```python
from build123d import *

# Parameters (mm, degrees)
F0_R     = 21
F0_R_2   = 0.8
F1_DEPTH = 5
F2_R     = 21
F3_DEPTH = 14
F4_R     = 21
F4_R_2   = 19
F5_DEPTH = 2.5
F6_SIZE  = 1


with BuildPart() as f1:
    # F0 (on Top) → F1 (new body)
    with BuildSketch(Plane.XY):
        Circle(F0_R)
        with Locations((-10, 0)):
            Circle(F0_R_2, mode=Mode.SUBTRACT)
        with BuildLine():
            Line((6, -6.5), (-6, -6.5))
            ThreePointArc((-6, -6.5), (-7.06066, -6.06066), (-7.5, -5))
            Line((-7.5, -5), (-7.5, 5))
            ThreePointArc((-7.5, 5), (-7.06066, 6.06066), (-6, 6.5))
            Line((-6, 6.5), (6, 6.5))
            ThreePointArc((6, 6.5), (7.06066, 6.06066), (7.5, 5))
            Line((7.5, 5), (7.5, -5))
            ThreePointArc((7.5, -5), (7.06066, -6.06066), (6, -6.5))
        make_face(mode=Mode.SUBTRACT)
        with Locations((10, 0)):
            Circle(F0_R_2, mode=Mode.SUBTRACT)
    extrude(amount=F1_DEPTH)

    # F2 (on face) → F3 (join)
    with BuildSketch(Plane.XY.offset(5)):
        Circle(F2_R)
        with BuildLine():
            Line((6, -6.5), (-6, -6.5))
            ThreePointArc((-6, -6.5), (-7.06066, -6.06066), (-7.5, -5))
            Line((-7.5, -5), (-7.5, 5))
            ThreePointArc((-7.5, 5), (-7.06066, 6.06066), (-6, 6.5))
            Line((-6, 6.5), (6, 6.5))
            ThreePointArc((6, 6.5), (7.06066, 6.06066), (7.5, 5))
            Line((7.5, 5), (7.5, -5))
            ThreePointArc((7.5, -5), (7.06066, -6.06066), (6, -6.5))
        make_face(mode=Mode.SUBTRACT)
    extrude(amount=F3_DEPTH)

    # F4 (on face) → F5 (join)
    with BuildSketch(Plane.XY.offset(19)):
        Circle(F4_R)
        Circle(F4_R_2, mode=Mode.SUBTRACT)
    extrude(amount=F5_DEPTH)

    # F6
    f6_edges = [f1.edges().sort_by_distance(p)[0] for p in [
        (-21, 0, 0),
    ]]
    chamfer(f6_edges, length=F6_SIZE)


solid = f1.part
```
For this review, take the finished solid that the model builds, in its own axes (mm). A direction names the side the tool comes from. Round coordinates to 2 decimals unless told otherwise and drop trailing zeros. Write each loop counter-clockwise with the first axis right and the second up, starting at its lowest first coordinate (ties: lowest second). Pieces come first, ordered by that corner, then holes. Notation, with made-up numbers: (74.5, 43.5) - (83.5, 43.5) arc R26 ccw to (83.5, 62.5) - close; hole circle Ø2 at (63.5, -34.5). An arc over 180 degrees is marked (long way). Answer as CSV lines item,"result". Start each with the question number.
(1) Add section A-A, the plane z = 12.5. State the section outline as (x, y) points.
(2) Mouldability with a two-part tool opening along X and no side actions: class faces 5 (the flat face through (0, -9, 0)), 6 (the cylindrical face through (-7.05, -6.07, 9.37)), 7 (the cylindrical face through (20.03, 6.31, 11.11)) as +X half, -X half, draft (parallel to the pull), parting line (faces both ways), or undercut.
(3) Add section C-C, the plane y = 0. State the section outline as (x, z) points.
(4) Add section B-B, the plane x = 0. State the section outline as (y, z) points, plus the area to 3 significant figures.
(5) For pin 1 (4 mm diameter, centred on x = 13.5, z = 8, fed in from +Y); pin 2 (19 mm diameter, centred on x = -8, y = 3.5, fed in from +Z); pin 3 (1.3 mm diameter, centred on x = -10, y = 0, fed in from -Z), all flat-tipped, find the tip position at first contact; note any pin that passes through.
(6) For line 1 (Y direction, x = 0, z = 20.3); line 2 (Y direction, x = 3, z = 3); line 3 (Z direction, x = 14.5, y = 7), list the stretches that pass through material, from the lowest coordinate up.
(7) Machinability: for faces 1 (the cylindrical face through (-7.07, 6.05, 9.37)), 2 (the flat face through (-10, 0, 5)), 3 (the cylindrical face through (8.767, -16.856, 20.232)), 4 (the flat face through (-16, -11, 21.5)), which of the approach directions +Z, -Z, +X, -X, +Y, -Y give a long, thin tool a straight path to every point of the face, cutting with its end or side? Answer none if there is none.
From the geometry:
1,outline,"circle Ø42 at (0, 0); hole (-7.5, -5) arc R1.5 ccw to (-6, -6.5) - (6, -6.5) arc R1.5 ccw to (7.5, -5) - (7.5, 5) arc R1.5 ccw to (6, 6.5) - (-6, 6.5) arc R1.5 ccw to (-7.5, 5) - close"
2,face 5,"draft"
2,face 6,"undercut"
2,face 7,"parting line"
3,outline,"(-21, 1) - (-20, 0) - (-10.8, 0) - (-10.8, 5) - (-9.2, 5) - (-9.2, 0) - (-7.5, 0) - (-7.5, 19) - (-19, 19) - (-19, 21.5) - (-21, 21.5) - close; (7.5, 0) - (9.2, 0) - (9.2, 5) - (10.8, 5) - (10.8, 0) - (20, 0) - (21, 1) - (21, 21.5) - (19, 21.5) - (19, 19) - (7.5, 19) - close"
4,outline,"(-21, 1) - (-20, 0) - (-6.5, 0) - (-6.5, 19) - (-19, 19) - (-19, 21.5) - (-21, 21.5) - close; (6.5, 0) - (20, 0) - (21, 1) - (21, 21.5) - (19, 21.5) - (19, 19) - (6.5, 19) - close"
4,area,"560 mm²"
5,pin 1,"stops at y = 17.57"
5,pin 2,"stops at z = 19"
5,pin 3,"stops at z = 5"
6,line 1,"y = -21 to -19, 19 to 21"
6,line 2,"y = -20.78 to -6.5, 6.5 to 20.78"
6,line 3,"z = 0 to 19"
7,face 1,"+Z, -Z"
7,face 2,"-Z"
7,face 3,"+Z"
7,face 4,"+Z, +X, -X, +Y, -Y"
